Here's how the part is built. I have some questions about the finished solid (model axes, mm). Face numbers are marked on the shaded views. A direction names the side the tool comes from. Coordinates: 2 decimals unless noted, no trailing zeros. Write each loop counter-clockwise with the first axis right and the second up, starting at its lowest first coordinate (ties: lowest second). Pieces come first, ordered by that corner, then holes.
(1) Please list where these lines run through material, in increasing order: probe 1 along Y at (x, z) = (0.6, 5); probe 2 along Y at (x, z) = (-2.05, 7); probe 3 along X at (y, z) = (2.75, 5.5).
(2) Imagine slicing it at A-A, the plane z = 3.5. List the corners of the cut face in (x, y) for me.
(3) Thinking about a two-plate mould opening in Z: for the marked faces 5, 6 and 7, which applies, released by +Z, released by -Z, zero draft, split by the parting line, or undercut?
(4) Which directions (+Z, -Z, +X, -X, +Y, -Y) give clear straight access to the entire face, cutting with the end or side of a thin tool? Please do the marked faces 1, 2, 3 and 4.
(5) For pin 1 Ø1.5 at (x, z) = (-1, 5.5) entering from -Y; pin 2 Ø1.5 at (x, z) = (-1, 2) entering from +Y, each with a flat end and sliding along its axis, tell me the tip position at first contact or that it passes through.
(6) Imagine slicing it at B-B, the plane y = 0. List the corners of the cut face in (x, z) for me, plus the area to 4 significant figures.
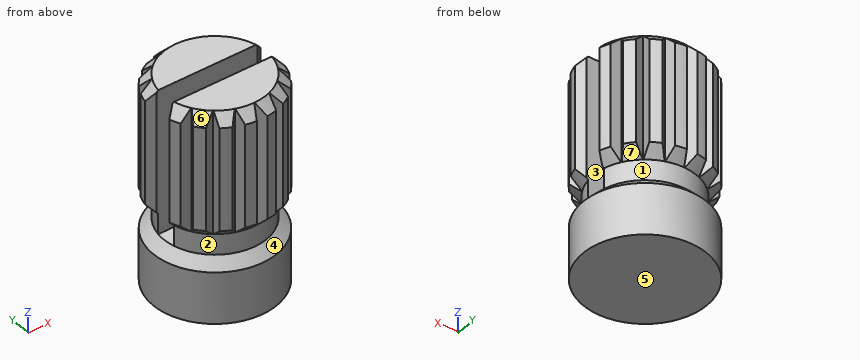
```python
from build123d import *

# Parameters (mm, degrees)
SKETCH_R           = 3
PAD_DEPTH          = 3
CHAMFER_SIZE       = 0.5
SKETCH001_R        = 2.5
PAD001_DEPTH       = 1
SKETCH002_R        = 3
PAD002_DEPTH       = 6
CHAMFER001_SIZE    = 0.499
CHAMFER002_SIZE    = 0.5
POCKET_DEPTH       = 6
POLARPATTERN_COUNT = 18
SKETCH004_W        = 7
SKETCH004_H        = 1
POCKET001_DEPTH    = 7


with BuildPart() as part:
    # Sketch → Pad (new body)
    with BuildSketch(Plane.XY):
        Circle(SKETCH_R)
    extrude(amount=PAD_DEPTH)

    # Chamfer
    chamfer_edges = [part.edges().sort_by_distance(p)[0] for p in [
        (-3, 0, 3),
    ]]
    chamfer(chamfer_edges, length=CHAMFER_SIZE)

    # Sketch001 → Pad001 (join)
    with BuildSketch(Plane.XY.offset(3)):
        Circle(SKETCH001_R)
    extrude(amount=PAD001_DEPTH)

    # Sketch002 → Pad002 (join)
    with BuildSketch(Plane.XY.offset(4)):
        Circle(SKETCH002_R)
    extrude(amount=PAD002_DEPTH)

    # Chamfer001
    chamfer001_edges = [part.edges().sort_by_distance(p)[0] for p in [
        (-3, 0, 4),
    ]]
    chamfer(chamfer001_edges, length=CHAMFER001_SIZE)

    # Chamfer002
    chamfer002_edges = [part.edges().sort_by_distance(p)[0] for p in [
        (-3, 0, 10),
    ]]
    chamfer(chamfer002_edges, length=CHAMFER002_SIZE)

    # Sketch003 → Pocket (cut)
    with BuildSketch(Plane.XY.offset(10)):
        with BuildLine():
            ThreePointArc((0.262071, 2.988531), (0.000606, 3), (-0.260863, 2.988637))
            Line((-0.260863, 2.988637), (0, 2.477175))
            Line((0, 2.477175), (0.262071, 2.988531))
        make_face()
    pocket = extrude(amount=-POCKET_DEPTH, mode=Mode.SUBTRACT)

    # PolarPattern: Pocket ×18 about axis
    polarpattern_axis = Axis((0, 0, 10), (0, 0, 1))
    for i in range(1, POLARPATTERN_COUNT):
        add(pocket.rotate(polarpattern_axis, i * 360 / POLARPATTERN_COUNT), mode=Mode.SUBTRACT)

    # Sketch004 → Pocket001 (cut)
    with BuildSketch(Plane.XY.offset(10)):
        Rectangle(SKETCH004_W, SKETCH004_H)
    extrude(amount=-POCKET001_DEPTH, mode=Mode.SUBTRACT)


solid = part.part
```
Recorded:
1. probe 1: y = -2.94 to -0.5, 0.5 to 2.94
1. probe 2: y = -2.09 to -0.5, 0.5 to 2.09
1. probe 3: x = -0.79 to -0.14, 0.14 to 0.8
2. outline: (-2.45, -0.5) arc R2.5 ccw to (2.45, -0.5) - close; (-2.45, 0.5) - (2.45, 0.5) arc R2.5 ccw to start
3. face 5: released by -Z
3. face 6: released by +Z
3. face 7: undercut
4. face 1: +Y
4. face 2: -Y
4. face 3: +Z, +X, -X
4. face 4: none
5. pin 1: stops at y = -2.99
5. pin 2: stops at y = 2.99
6. outline: (-3, 0) - (3, 0) - (3, 2.5) - (2.5, 3) - (-2.5, 3) - (-3, 2.5) - close
6. area: 17.75 mm2
